Could you check a few things on this model? Use its own coordinates, in mm. Coordinates: 2 decimals unless noted, no trailing zeros. Loops run counter-clockwise (first coordinate to the right, second up) from the corner with the lowest first, then second, coordinate; pieces in that order, holes last. Notation, with made-up numbers: M 17.25,52.25 L 51.25,52.25 A23 cw 51.25,67.25 Z; hole C -33.75,-18.75 d1. An arc over 180 degrees is marked long. Write each question's results on one line, items separated by ' | '.
```python
from build123d import *

# Parameters (mm, degrees)
SKETCH1_W           = 31
SKETCH1_H           = 25
SKETCH1_R           = 1.45
BOSS_EXTRUDE1_DEPTH = 13
SKETCH2_W           = 20
SKETCH2_H           = 12
CUT_EXTRUDE1_DEPTH  = 0.2
CUT_EXTRUDE2_DEPTH  = 14
FILLET1_R           = 1


with BuildPart() as part:
    # Sketch1 → Boss-Extrude1 (new body)
    with BuildSketch(Plane(origin=(0, 0, 0), x_dir=(1, 0, 0), z_dir=(0, 1, 0))):
        with Locations((0, -1.439483729)):
            Rectangle(SKETCH1_W, SKETCH1_H)
        with Locations((-11.5, -9.939483729)):
            Circle(SKETCH1_R, mode=Mode.SUBTRACT)
        with Locations((11.5, -9.939483729)):
            Circle(SKETCH1_R, mode=Mode.SUBTRACT)
    extrude(amount=BOSS_EXTRUDE1_DEPTH)

    # Sketch2 → Cut-Extrude1 (cut)
    with BuildSketch(Plane.XY.offset(13.939483729)):
        with Locations((0, 6.5)):
            Rectangle(SKETCH2_W, SKETCH2_H)
    extrude(amount=-CUT_EXTRUDE1_DEPTH, mode=Mode.SUBTRACT)

    # Sketch3 → Cut-Extrude2 (cut, through all)
    with BuildSketch(Plane(origin=(0, 13, 0), x_dir=(1, 0, 0), z_dir=(0, 1, 0))):
        Polygon((-15.5, 4.060516271), (-3.375644347, 11.060516271), (-15.5, 11.060516271), align=None)
    extrude(amount=-CUT_EXTRUDE2_DEPTH, mode=Mode.SUBTRACT)

    # Fillet1
    fillet1_edges = [part.edges().sort_by_distance(p)[0] for p in [
        (15.5, 6.5, 13.939483729),
        (-15.5, 6.5, 13.939483729),
        (15.5, 6.5, -11.060516271),
    ]]
    fillet(fillet1_edges, radius=FILLET1_R)


solid = part.part
```
(1) Imagine slicing it at B-B, the plane y = 7.5. List the corners of the cut face in (x, z) for me.
Reported:
outline: M -15.5,-4.06 L -3.38,-11.06 L 14.5,-11.06 A1 ccw 15.5,-10.06 L 15.5,12.94 A1 ccw 14.5,13.94 L 10,13.94 L 10,13.74 L -10,13.74 L -10,13.94 L -14.5,13.94 A1 ccw -15.5,12.94 Z; hole C -11.5,9.94 d2.9; hole C 11.5,9.94 d2.9
(2) Imagine slicing it at D-D, the plane z = -5.25. List the corners of the cut face in (x, y) for me, and give its area (3 significant figures).
Reported:
outline: M -13.44,0 L 15.5,0 L 15.5,13 L -13.44,13 Z | area: 376 mm2
(3) If we mould it in two halves opening along Y, with no side actions, what happens to faces 1 (the cylindrical face through (-12.95, 6.41, 9.88)), 2 (the flat face through (0, 7, 13.739)), 3 (the flat face through (0, 13, 1))? For each: released by +Y, released by -Y, zero draft, split by the parting line, or undercut.
Reported:
face 1: zero draft | face 2: undercut | face 3: released by +Y
(4) Please list where these lines run through material, in increasing order: probe 1 along Z at (x, y) = (11.5, 6.25); probe 2 along Z at (x, y) = (0, 6.5); probe 3 along Z at (x, y) = (-11.5, 2.5). Write a range as from..to.
Reported:
probe 1: z = -11.06..8.49, 11.39..13.94 | probe 2: z = -11.06..13.74 | probe 3: z = -6.37..8.49, 11.39..13.94
(5) Imagine slicing it at A-A, the plane x = 11.5. List the corners of the cut face in (y, z) for me, and give its area (3 significant figures).
Reported:
outline: M 0,-11.06 L 13,-11.06 L 13,8.49 L 0,8.49 Z; M 0,11.39 L 13,11.39 L 13,13.94 L 0,13.94 Z | area: 287 mm2
(6) Imagine slicing it at C-C, the plane x = -9. List the corners of the cut face in (y, z) for me.
Reported:
outline: M 0,-7.81 L 13,-7.81 L 13,13.94 L 12.5,13.94 L 12.5,13.74 L 0.5,13.74 L 0.5,13.94 L 0,13.94 Z
(7) Will this pin go through, and if not, where does the flat tip stop? P1, Ø2.5, axis at x = 11.5, z = 9.94, coming from the -Y side.
Reported:
P1: passes through
